The model under review builds one solid part; all positions refer to its coordinate system, in mm. Round coordinates to 2 decimals unless told otherwise and drop trailing zeros. Order: outer loops, then holes, each group sorted by start corner. A loop starts at its lowest first (then second) coordinate and runs counter-clockwise, first axis right, second up. Notation, with made-up numbers: (-7, 35.25) -> (9, 35.25) arc R17 cw to (9, 65.25) -> close; hole circle Ø7 at (2, 68). An arc over 180 degrees is marked (long way). Use a Markdown table: item, result. Add a question column.
```python
from build123d import *

# Parameters (mm, degrees)
BOSS_EXTRUDE1_DEPTH = 210.295833075
CUT_EXTRUDE3_DEPTH  = 2024.344561921
BOSS_EXTRUDE2_DEPTH = 77
SKETCH7_W           = 5
SKETCH7_H           = 30
BOSS_EXTRUDE4_DEPTH = 25.5


with BuildPart() as part:
    # Sketch2 → Boss-Extrude1 (new body)
    with BuildSketch(Plane.XY.offset(116.791940296)):
        Polygon((-1177.651750867, 1643.980030656), (-1173.163691186, 1646.183963573), (-1041.945008983, 1378.971984434), (-1046.433068663, 1376.768051516), align=None)
    extrude(amount=BOSS_EXTRUDE1_DEPTH)

    # Sketch5 → Cut-Extrude3 (cut, through all)
    with BuildSketch(Plane(origin=(-293.905010595, -144.326718837, 0), x_dir=(0, 0, 1), z_dir=(-0.8976119360459706, -0.4407865835841701, 0))):
        Polygon((132.47954497, 1831.677464024), (116.791940296, 1831.677464024), (116.791940296, 1994.749190054), (327.087773371, 1994.749190054), (327.087773371, 1623.434080327), (116.791940296, 1623.434080327), (116.791940296, 1779.483651489), (162.291940296, 1779.483651489), (162.291940296, 1711.327604599), (182.291940296, 1711.327604599), (182.291940296, 1778.260209904), align=None)
    extrude(amount=CUT_EXTRUDE3_DEPTH, mode=Mode.SUBTRACT)

    # Sketch6 → Boss-Extrude2 (add)
    with BuildSketch(Plane(origin=(0, 0, 116.791940296), x_dir=(-1, 0, 0), z_dir=(0, 0, -1))):
        Polygon((1087.597149779, 1460.594038789), (1083.109090099, 1462.797971707), (1172.730720222, 1645.302267261), (1177.218779902, 1643.098334343), align=None)
    extrude(amount=BOSS_EXTRUDE2_DEPTH)

    # Sketch7 → Boss-Extrude4 (add)
    with BuildSketch(Plane(origin=(-789.204079504, 1607.124690544, 0), x_dir=(0.8976119360459841, 0.44078658358414263, 0), z_dir=(0.44078658358414263, -0.8976119360459841, 0))):
        with Locations((-329.92992689, 54.791940296)):
            Rectangle(SKETCH7_W, SKETCH7_H)
    extrude(amount=BOSS_EXTRUDE4_DEPTH)


solid = part.part
```
Q1. Add section C-C, the plane z = 65.5. Give the boundary of the cut face in (x, y), then the cut area to 3 significant figures.
Q2. Draft analysis for pull direction Z (two halves, no side actions). For faces 1 (the face through (-1080, 1450, 69.792)), 2 (the face through (-1125, 1543, 39.792)), 3 (the face through (-1065, 1420, 182.292)), state which applies: released by +Z, released by -Z, zero draft, split by the parting line, or undercut.
Q3. Add section B-B, the plane y = 1616. Give the boundary of the cut face in (x, z).
Q4. For pin 1 (23 mm diameter, centred on x = -1143.5, y = 1556.5, fed in from +Z); pin 2 (10 mm diameter, centred on x = -1104, z = 85.5, fed in from -Y); pin 3 (5 mm diameter, centred on y = 1461.5, z = 91.5, fed in from -X); pin 4 (1 mm diameter, centred on x = -1078, y = 1436, fed in from +Z), all flat-tipped, find the tip position at first contact; note any pin that passes through.
Q5. Add section A-A, the plane z = 101. Give the boundary of the cut face in (x, y), then the cut area to 3 significant figures.
Q6. To check wall thickness, follow line 1 along Z through (x, y) = (-1106, 1503); line 2 along X through (y, z) = (1536, 113.5); line 3 along Y through (x, z) = (-1108, 51.5). State the ranges of each line that lie inside material, in increasing order.
Return value:
| question | item | result |
|---|---|---|
| 1 | outline | (-1177.22, 1643.1) -> (-1076.36, 1437.7) -> (-1071.87, 1439.91) -> (-1172.73, 1645.3) -> close |
| 1 | area | 1,140 mm² |
| 2 | face 1 | undercut |
| 2 | face 2 | released by -Z |
| 2 | face 3 | released by +Z |
| 3 | outline | (-1163.91, 39.79) -> (-1158.34, 39.79) -> (-1158.34, 116.79) -> (-1163.91, 116.79) -> close |
| 4 | pin 1 | z = 116.79 |
| 4 | pin 2 | y = 1483.81 |
| 4 | pin 3 | x = -1089.27 |
| 4 | pin 4 | through |
| 5 | outline | (-1177.22, 1643.1) -> (-1087.6, 1460.59) -> (-1083.11, 1462.8) -> (-1172.73, 1645.3) -> close |
| 5 | area | 1,020 mm² |
| 6 | line 1 | 39.79 to 116.79 |
| 6 | line 2 | -1124.63 to -1119.06 |
| 6 | line 3 | 1502.14 to 1513.49 |
